Answer from the drawing. Dimensions are ordinates in mm from the lowest x, y and z of the part. Round coordinates to 2 decimals unless told otherwise and drop trailing zeros. Write each loop counter-clockwise with the first axis right and the second up, starting at its lowest first coordinate (ties: lowest second). Pieces come first, ordered by that corner, then holes. Notation, with made-up numbers: (70, 5) - (118, 5) arc R12 ccw to (118, 28) - close; hole circle Ø2 at (89.5, -19.5). An arc over 180 degrees is marked (long way). Answer as CSV lines item,"result". Start each with the question number.
1) Find section B-B on x = 50. Determine the outline of the cut face in (y, z), then the cut area to 3 significant figures.
2) Find section D-D on y = 9.5. Determine the outline of the cut face in (x, z).
3) Each of these flat-tipped pins is pushed along its axis until it touches: pin 1 (5 mm diameter, centred on x = 15, y = 25, fed in from +Z); pin 2 (1.5 mm diameter, centred on x = 97, z = 1, fed in from -Y) (3 decimals); pin 3 (0.9 mm diameter, centred on x = 54, z = 1.5, fed in from -Y); pin 4 (0.9 mm diameter, centred on y = 2, z = 1.5, fed in from -X). Where does it stop, or does it pass through?
4) Find section A-A on y = 25. Determine the outline of the cut face in (x, z).
5) Consider line 1 along Y through (x, z) = (15, 0.65); line 2 along X through (y, z) = (3.5, 0.8); line 3 along Y through (x, z) = (50, 1.5). Determine where each line is inside the solid, lowest interval first.
6) Find section C-C on x = 15. Determine the outline of the cut face in (y, z), then the cut area to 3 significant figures.
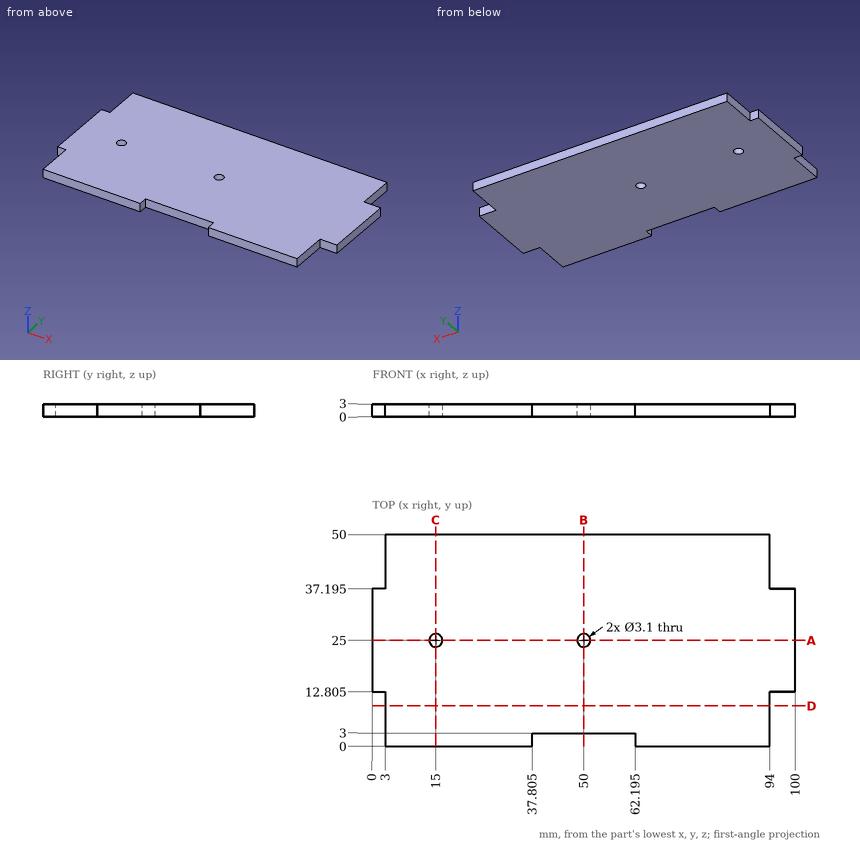
Check values:
1,outline,"(3, 0) - (23.45, 0) - (23.45, 3) - (3, 3) - close; (26.55, 0) - (50, 0) - (50, 3) - (26.55, 3) - close"
1,area,"132 mm^2"
2,outline,"(3, 0) - (94, 0) - (94, 3) - (3, 3) - close"
3,pin 1,"stops at z = 3"
3,pin 2,"stops at y = 12.805"
3,pin 3,"stops at y = 3"
3,pin 4,"stops at x = 3"
4,outline,"(0, 0) - (13.45, 0) - (13.45, 3) - (0, 3) - close; (16.55, 0) - (48.45, 0) - (48.45, 3) - (16.55, 3) - close; (51.55, 0) - (100, 0) - (100, 3) - (51.55, 3) - close"
5,line 1,"y = 0 to 23.45, 26.55 to 50"
5,line 2,"x = 3 to 94"
5,line 3,"y = 3 to 23.45, 26.55 to 50"
6,outline,"(0, 0) - (23.45, 0) - (23.45, 3) - (0, 3) - close; (26.55, 0) - (50, 0) - (50, 3) - (26.55, 3) - close"
6,area,"141 mm^2"
